from build123d import *

# Parameters (mm, degrees)
BASE_FLANGE1_DEPTH = 3.175
FILLET1_R          = 20
SKETCH2_R          = 2.5
CUT_EXTRUDE1_DEPTH = 10


# Sheet-metal steps are written as plain solids
with BuildPart() as part:
    # Sketch1 → Base-Flange1 (new body)
    with BuildSketch(Plane(origin=(0, 0, 0), x_dir=(0, 0, -1), z_dir=(1, 0, 0))):
        Polygon((0, 0), (-25.767161182, 294.52), (375.792838818, 294.52), (350.025677637, 0), align=None)
    extrude(amount=-BASE_FLANGE1_DEPTH)

    # Fillet1
    fillet1_edges = [part.edges().sort_by_distance(p)[0] for p in [
        (-1.5875, 0, 0),
        (-1.5875, 294.52, 25.767161182),
        (-1.5875, 294.52, -375.792838818),
        (-1.5875, 0, -350.025677637),
    ]]
    fillet(fillet1_edges, radius=FILLET1_R)

    # Sketch2 → Cut-Extrude1 (cut)
    with BuildSketch(Plane(origin=(0, 0, 0), x_dir=(0, 0, -1), z_dir=(1, 0, 0))):
        with Locations((46.113408302, 274.52)):
            Circle(SKETCH2_R)
        with Locations((303.890562759, 274.52)):
            Circle(SKETCH2_R)
        with Locations((48.402729519, 21.11878104)):
            Circle(SKETCH2_R)
        with Locations((301.622948118, 21.11878104)):
            Circle(SKETCH2_R)
    extrude(amount=-CUT_EXTRUDE1_DEPTH, mode=Mode.SUBTRACT)


solid = part.part
Geometry: final body of the model. Coordinates: model frame, mm. Round coordinates to 2 decimals unless told otherwise and drop trailing zeros. Loops run counter-clockwise (first coordinate to the right, second up) from the corner with the lowest first, then second, coordinate; pieces in that order, holes last. Notation, with made-up numbers: (21.5, 26.25) - (65.5, 26.25) arc R36 ccw to (65.5, 63.25) - close; hole circle Ø9 at (-35, -17). An arc over 180 degrees is marked (long way). Write each question's results on one line, items separated by ' | '. Start each with the question number.
1) First-contact query: P1, Ø4, axis at y = 21.12, z = -48.4, coming from the +X side; P2, Ø1, axis at x = -0.5, y = 248, coming from the -Z side. Flat tips, straight axial feed; report the tip coordinate or a pass-through.
2) Line query: probe 1 along Z at (x, y) = (-2.05, 274.52); probe 2 along Z at (x, y) = (-2.4, 275.5); probe 3 along Y at (x, z) = (-1.95, -303.5). Output: solid intervals per line, ascending. Write a range as [from, to].
3) Cut plane B-B on y = 114. Return loops of the section in (x, z) (3 decimals), then the cut area to 3 significant figures.
4) Cut plane C-C on y = 166.5. Return loops of the section in (x, z) (3 decimals).
5) Cut plane A-A on x = -0.65. Return loops of the section in (y, z), then the cut area to 3 significant figures.
Verdict:
1) P1: passes through | P2: stops at z = -371.77
2) probe 1: z = [-373.97, -306.39], [-301.39, -48.61], [-43.61, 23.94] | probe 2: z = [-373.94, -306.19], [-301.59, -48.41], [-43.81, 23.92] | probe 3: y = [0, 19.47], [22.77, 272.05], [276.99, 294.52]
3) outline: (-3.175, -359.999) - (0, -359.999) - (0, 9.974) - (-3.175, 9.974) - close | area: 1,170 mm2
4) outline: (-3.175, -364.593) - (0, -364.593) - (0, 14.567) - (-3.175, 14.567) - close
5) outline: (0, -331.7) arc R20 ccw to (18.26, -351.62) - (272.78, -373.89) arc R20 ccw to (294.52, -353.97) - (294.52, 3.94) arc R20 ccw to (272.78, 23.86) - (18.26, 1.6) arc R20 ccw to (0, -18.33) - close; hole circle Ø5 at (21.12, -301.62); hole circle Ø5 at (21.12, -48.4); hole circle Ø5 at (274.52, -303.89); hole circle Ø5 at (274.52, -46.11) | area: 110,000 mm2
